For this review, take the finished solid that the model builds, in its own axes (mm). A direction names the side the tool comes from. Coordinates: 2 decimals unless noted, no trailing zeros. Order: outer loops, then holes, each group sorted by start corner. A loop starts at its lowest first (then second) coordinate and runs counter-clockwise, first axis right, second up. Notation, with made-up numbers: M 82,85.5 L 118,85.5 A14 ccw 118,101.5 Z; hole C 65,-20.5 d4. An arc over 180 degrees is marked long. Use CSV: the item, a comma, the result in double quotes.
```python
from build123d import *

# Parameters (mm, degrees)
SKETCH1_W           = 30
SKETCH1_H           = 26.5
SKETCH1_R           = 5
SKETCH1_R_2         = 1.5
BOSS_EXTRUDE1_DEPTH = 3
SKETCH2_W           = 3
SKETCH2_H           = 26.5
BOSS_EXTRUDE2_DEPTH = 33
CUT_EXTRUDE1_DEPTH  = 33
SKETCH4_R           = 5
CUT_EXTRUDE2_DEPTH  = 49.513529041


with BuildPart() as part:
    # Sketch1 → Boss-Extrude1 (new body)
    with BuildSketch(Plane(origin=(0, 0, 0), x_dir=(1, 0, 0), z_dir=(0, 1, 0))):
        Rectangle(SKETCH1_W, SKETCH1_H)
        with Locations(Location((0, 0, 0), (0, 0, 270))):
            Circle(SKETCH1_R, mode=Mode.SUBTRACT)
        with Locations(Location((7.5, 8.25, 0), (0, 0, 270))):
            Circle(SKETCH1_R_2, mode=Mode.SUBTRACT)
        with Locations(Location((-7.5, 8.25, 0), (0, 0, 90))):
            Circle(SKETCH1_R_2, mode=Mode.SUBTRACT)
        with Locations(Location((-7.5, -8.25, 0), (0, 0, 270))):
            Circle(SKETCH1_R_2, mode=Mode.SUBTRACT)
        with Locations(Location((7.5, -8.25, 0), (0, 0, 90))):
            Circle(SKETCH1_R_2, mode=Mode.SUBTRACT)
    extrude(amount=BOSS_EXTRUDE1_DEPTH)

    # Sketch2 → Boss-Extrude2 (add)
    with BuildSketch(Plane(origin=(0, 0, 0), x_dir=(1, 0, 0), z_dir=(0, 1, 0))):
        with Locations((16.5, 0)):
            Rectangle(SKETCH2_W, SKETCH2_H)
    extrude(amount=BOSS_EXTRUDE2_DEPTH)

    # Sketch3 → Cut-Extrude1 (cut)
    with BuildSketch(Plane.ZY.offset(-15)):
        with BuildLine():
            Line((0, 33), (-13.25, 33))
            Line((-13.25, 33), (-13.25, 19.75))
            ThreePointArc((-13.25, 19.75), (-9.369164851, 29.119164851), (0, 33))
        make_face()
        with BuildLine():
            Line((13.25, 33), (0, 33))
            ThreePointArc((0, 33), (9.369164851, 29.119164851), (13.25, 19.75))
            Line((13.25, 19.75), (13.25, 33))
        make_face()
    extrude(amount=-CUT_EXTRUDE1_DEPTH, mode=Mode.SUBTRACT)

    # Sketch4 → Cut-Extrude2 (cut, through all)
    with BuildSketch(Plane(origin=(18, 0, 0), x_dir=(0, 0, -1), z_dir=(1, 0, 0))):
        with Locations((0, 19.75)):
            Circle(SKETCH4_R)
    extrude(amount=-CUT_EXTRUDE2_DEPTH, mode=Mode.SUBTRACT)


solid = part.part
```
Item 1: Add section C-C on x = 7.5. State the section outline as (y, z) points, and give its area (3 significant figures).
Solutions:
outline,"M 0,-13.25 L 3,-13.25 L 3,-9.75 L 0,-9.75 Z; M 0,-6.75 L 3,-6.75 L 3,6.75 L 0,6.75 Z; M 0,9.75 L 3,9.75 L 3,13.25 L 0,13.25 Z"
area,"61.5 mm^2"
Item 2: Add section B-B on z = -7.5. State the section outline as (x, y) points, and give its area (3 significant figures).
Solutions:
outline,"M -15,0 L -8.8,0 L -8.8,3 L -15,3 Z; M -6.2,0 L 6.2,0 L 6.2,3 L -6.2,3 Z; M 8.8,0 L 18,0 L 18,30.67 L 15,30.67 L 15,3 L 8.8,3 Z"
area,"166 mm^2"
Item 3: Add section A-A on x = 0. State the section outline as (y, z) points, and give its area (3 significant figures).
Solutions:
outline,"M 0,-13.25 L 3,-13.25 L 3,-5 L 0,-5 Z; M 0,5 L 3,5 L 3,13.25 L 0,13.25 Z"
area,"49.5 mm^2"
Item 4: Draft analysis for pull direction Y (two halves, no side actions). For faces 1 (the face through (18, 13, 0)), 2 (the face through (0, 3, -6)), 3 (the face through (16.52, 14.87, 1.08)), 4 (the face through (5, 0, -3)), state which applies: released by +Y, released by -Y, zero draft, split by the parting line, or undercut.
Solutions:
face 1,"zero draft"
face 2,"released by +Y"
face 3,"undercut"
face 4,"released by -Y"
Item 5: To check wall thickness, follow line 1 along X through (y, z) = (0.85, 8.25); line 2 along Z through (x, y) = (-7, 1); line 3 along Y through (x, z) = (14.5, -2.75). State the ranges of each line that lie inside material, in increasing order. Write a range as [from, to].
Solutions:
line 1,"[-15, -9], [-6, 6], [9, 18]"
line 2,"[-13.25, -9.66], [-6.84, 6.84], [9.66, 13.25]"
line 3,"[0, 3]"
Item 6: For faces 5 (the face through (-6.036, 1.479, -7.925)), 6 (the face through (15, 14, 0)), list the 3-axis set-ups (+Z, -Z, +X, -X, +Y, -Y) from which the entire face can be reached by the end or side of a thin tool; tool diameter is ignored.
Solutions:
face 5,"+Y, -Y"
face 6,"+Z, -Z, -X, +Y"
Item 7: Clearance check with flat-ended pins moving along their axes: pin 1 Ø2.5 at (x, z) = (7.5, 8.25) entering from +Y; pin 2 Ø3 at (x, z) = (5.5, -2) entering from -Y; pin 3 Ø6 at (y, z) = (20.5, 3.5) entering from -X; pin 4 Ø5 at (x, z) = (1, 5.5) entering from +Y. State where each tip first meets the part, or that it passes through.
Solutions:
pin 1,"through"
pin 2,"y = 0"
pin 3,"x = 15"
pin 4,"y = 3"
Item 8: Add section D-D on y = 17.5. State the section outline as (x, z) points.
Solutions:
outline,"M 15,-13.25 L 18,-13.25 L 18,-4.47 L 15,-4.47 Z; M 15,4.47 L 18,4.47 L 18,13.25 L 15,13.25 Z"
